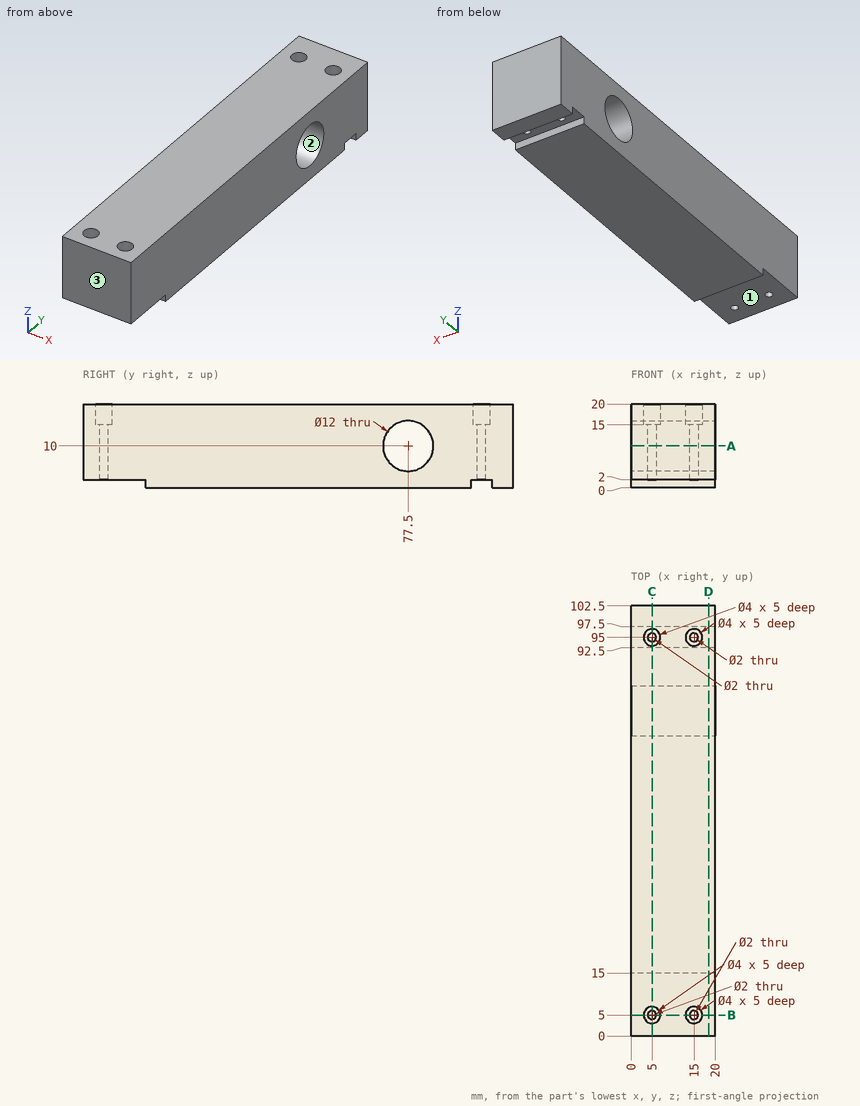
Drawing for the job (mm, zero at the part's lowest x, y, z). Round coordinates to 2 decimals unless told otherwise and drop trailing zeros. Order: outer loops, then holes, each group sorted by start corner. A loop starts at its lowest first (then second) coordinate and runs counter-clockwise, first axis right, second up. Notation, with made-up numbers: M -10,88.25 L 6,88.25 A10 cw 6,106.25 Z; hole C 26,-23.75 d7. An arc over 180 degrees is marked long. Use one line per item in the form item = value.
Q1. Saw through at D-D on x = 18.5. Give the cut face in (y, z), then the cut area to 3 significant figures.
Recorded:
outline = M 0,2 L 15,2 L 15,0 L 92.5,0 L 92.5,2 L 97.5,2 L 97.5,0 L 102.5,0 L 102.5,20 L 0,20 Z; hole C 77.5,10 d12
area = 1,900 mm^2
Q2. Flat gauge pins, fed straight in: P1, Ø2, axis at x = 14.5, y = 95, coming from the +Z side; P2, Ø7, axis at y = 77.5, z = 10, coming from the +X side; P3, Ø3, axis at x = 15, y = 95, coming from the -Z side; P4, Ø1, axis at x = 5.5, z = 1, coming from the -Y side. Where does each tip first touch, or does it go through?
Recorded:
P1 = 15
P2 = through
P3 = 2
P4 = 15
Q3. Saw through at C-C on x = 5. Give the cut face in (y, z).
Recorded:
outline = M 0,2 L 4,2 L 4,15 L 3,15 L 3,20 L 0,20 Z; M 6,2 L 15,2 L 15,0 L 92.5,0 L 92.5,2 L 94,2 L 94,15 L 93,15 L 93,20 L 7,20 L 7,15 L 6,15 Z; M 96,2 L 97.5,2 L 97.5,0 L 102.5,0 L 102.5,20 L 97,20 L 97,15 L 96,15 Z; hole C 77.5,10 d12
Q4. Saw through at B-B on y = 5. Give the cut face in (x, z).
Recorded:
outline = M 0,2 L 4,2 L 4,15 L 3,15 L 3,20 L 0,20 Z; M 6,2 L 14,2 L 14,15 L 13,15 L 13,20 L 7,20 L 7,15 L 6,15 Z; M 16,2 L 20,2 L 20,20 L 17,20 L 17,15 L 16,15 Z
Q5. Probe L1, parallel to Y at x = 15, z = 18.65; L2, parallel to X at y = 95, z = 18; L3, parallel to X at y = 95, z = 5. List the from-to ranges inside material, lowest first.
Recorded:
L1 = 0 to 3, 7 to 93, 97 to 102.5
L2 = 0 to 3, 7 to 13, 17 to 20
L3 = 0 to 4, 6 to 14, 16 to 20
Q6. Saw through at A-A on z = 10. Give the cut face in (x, y), then the cut area to 3 significant figures.
Recorded:
outline = M 0,0 L 20,0 L 20,71.5 L 0,71.5 Z; M 0,83.5 L 20,83.5 L 20,102.5 L 0,102.5 Z; hole C 5,5 d2; hole C 5,95 d2; hole C 15,5 d2; hole C 15,95 d2
area = 1,800 mm^2
Q7. Two-plate mould, pull along Z, no slides. Class the marked faces 1, 2 and 3: +Z half, -Z half, draft (parallel to the pull), parting line (faces both ways), or undercut.
Recorded:
face_1 = -Z half
face_2 = undercut
face_3 = draft
